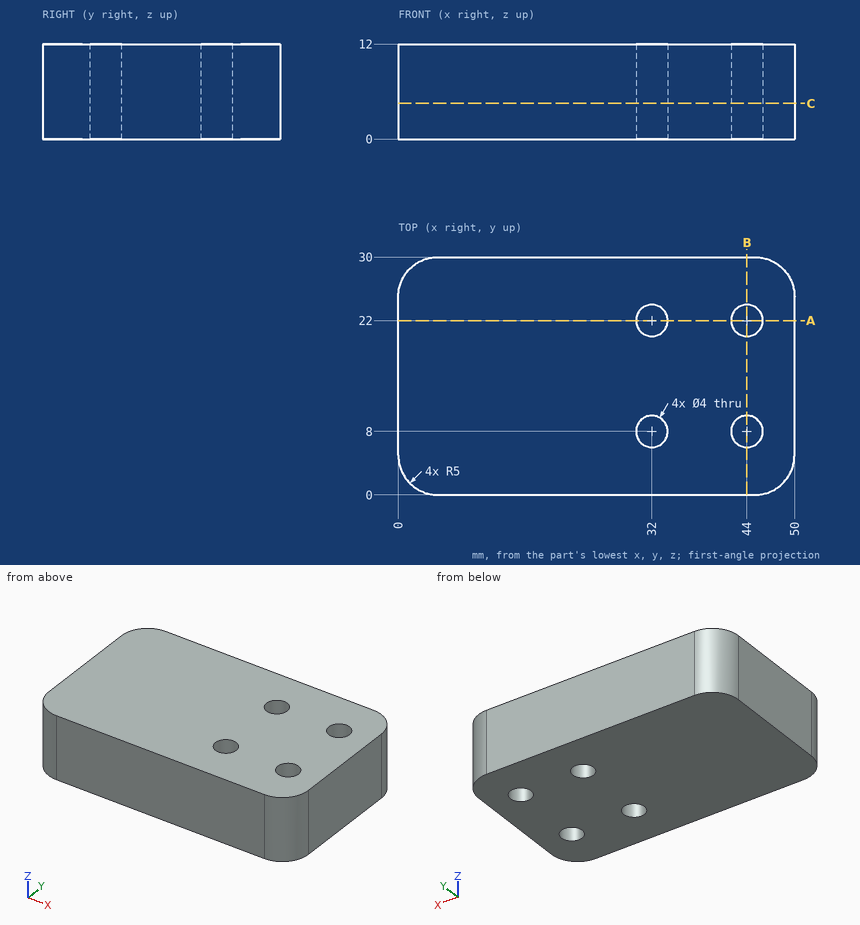
Could you check a few things on this drawing? It's one solid part, dimensions in mm from its lowest x, y, z. Give positions to 0.01 mm unless a question says otherwise; leave off trailing zeros. Loops run counter-clockwise (first coordinate to the right, second up) from the corner with the lowest first, then second, coordinate; pieces in that order, holes last. Notation, with made-up numbers: (72.25, -23) -> (89.25, -23) arc R23 cw to (89.25, 13) -> close; hole circle Ø5 at (-9, 38.25). An arc over 180 degrees is marked (long way). Answer as CSV lines item,"result". Start each with the question number.
(1) If we section it at B-B on x = 44: Write out the boundary of the cut face in (y, z).
(2) If we section it at C-C on z = 4.5: Write out the boundary of the cut face in (x, y), then the cut area to 3 significant figures.
(3) If we section it at A-A on y = 22: Write out the boundary of the cut face in (x, z), then the cut area to 3 significant figures.
(4) I need wall thicknesses on probe 1 along Y at (x, z) = (43, 9); probe 2 along Y at (x, z) = (42.5, 7.5); probe 3 along X at (y, z) = (22.75, 1.75). Which ranges of each line are inside material? Lowest first, please.
Computed:
1,outline,"(0, 0) -> (6, 0) -> (6, 12) -> (0, 12) -> close; (10, 0) -> (20, 0) -> (20, 12) -> (10, 12) -> close; (24, 0) -> (30, 0) -> (30, 12) -> (24, 12) -> close"
2,outline,"(0, 5) arc R5 ccw to (5, 0) -> (45, 0) arc R5 ccw to (50, 5) -> (50, 25) arc R5 ccw to (45, 30) -> (5, 30) arc R5 ccw to (0, 25) -> close; hole circle Ø4 at (32, 8); hole circle Ø4 at (32, 22); hole circle Ø4 at (44, 8); hole circle Ø4 at (44, 22)"
2,area,"1,430 mm2"
3,outline,"(0, 0) -> (30, 0) -> (30, 12) -> (0, 12) -> close; (34, 0) -> (42, 0) -> (42, 12) -> (34, 12) -> close; (46, 0) -> (50, 0) -> (50, 12) -> (46, 12) -> close"
3,area,"504 mm2"
4,probe 1,"y = 0 to 6.27, 9.73 to 20.27, 23.73 to 30"
4,probe 2,"y = 0 to 6.68, 9.32 to 20.68, 23.32 to 30"
4,probe 3,"x = 0 to 30.15, 33.85 to 42.15, 45.85 to 50"
